from build123d import *

# Parameters (mm, degrees)
F0_R     = 10
F1_DEPTH = 25
F3_DEPTH = 12
F5_DEPTH = 25


with BuildPart() as f1:
    # F0 (on Top) → F1 (new body)
    with BuildSketch(Plane.XY):
        Circle(F0_R)
    extrude(amount=F1_DEPTH)

    # F2 (on face) → F3 (cut)
    with BuildSketch(Plane.XY.offset(25)):
        Polygon((2.886751, 5), (-2.886751, 5), (-5.773503, 0), (-2.886751, -5), (2.886751, -5), (5.773503, 0), align=None)
    extrude(amount=-F3_DEPTH, mode=Mode.SUBTRACT)

    # F4 (on face) → F5 (cut)
    with BuildSketch(Plane(origin=(0, 0, 0), x_dir=(1, 0, 0), z_dir=(0, 0, -1))):
        Polygon((1.057785, -4.400124), (4.400124, 1.057785), (-1.057785, 4.400124), (-4.400124, -1.057785), align=None)
    extrude(amount=-F5_DEPTH, mode=Mode.SUBTRACT)


solid = f1.part
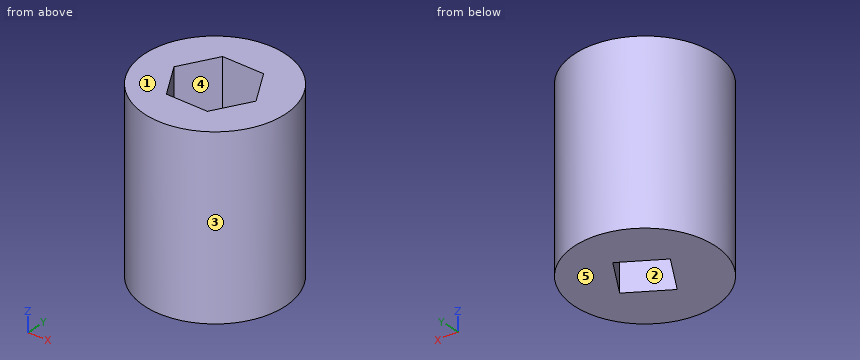
Work out the finished part from the listing and answer in its coordinate system (mm). Face numbers are marked on the shaded views. A direction names the side the tool comes from. Coordinates: 2 decimals unless noted, no trailing zeros. Write each loop counter-clockwise with the first axis right and the second up, starting at its lowest first coordinate (ties: lowest second). Pieces come first, ordered by that corner, then holes. Notation, with made-up numbers: (-8, 28.25) - (-2, 28.25) arc R22 cw to (-2, 59.25) - close; hole circle Ø5 at (-34.5, 89). An arc over 180 degrees is marked (long way). One line per question, with ' | ' between items.
1) For the marked faces 4 and 5, determine the directions among +Z, -Z, +X, -X, +Y, -Y from which every point of the face is accessible in a straight line to the end or side of a thin tool.
Checks:
face 4: +Z | face 5: -Z, +X, -X, +Y, -Y
2) Flat-ended cylindrical pins translate along their axes: P1, Ø1.5, axis at x = 2, z = 14, coming from the +Y side; P2, Ø2, axis at x = 7.5, z = 20, coming from the -Y side; P3, Ø10, axis at y = 5.5, z = 7, coming from the +X side. Find the tip coordinate at first contact, or state that the pin passes through.
Checks:
P1: y = 9.92 | P2: y = -7.6 | P3: x = 9.99
3) Consider probe 1 along Y at (x, z) = (-4.25, 3.75); probe 2 along X at (y, z) = (4, 10.75); probe 3 along X at (y, z) = (1.75, 8.75). Determine where each line is inside the solid, lowest interval first. Write a range as [from, to].
Checks:
probe 1: [-9.05, 0.81], [1.15, 9.05] | probe 2: [-9.17, 0.4], [1.3, 9.17] | probe 3: [-9.85, -3.27], [2.68, 9.85]
4) Find section D-D, the plane x = -5.25. Determine the outline of the cut face in (y, z).
Checks:
outline: (-8.51, 0) - (8.51, 0) - (8.51, 25) - (0.91, 25) - (0.91, 13) - (-0.91, 13) - (-0.91, 25) - (-8.51, 25) - close
5) Find section B-B, the plane z = 7.75. Determine the outline of the cut face in (x, y).
Checks:
outline: circle Ø20 at (0, 0); hole (-4.4, 1.06) - (-1.06, -4.4) - (4.4, -1.06) - (1.06, 4.4) - close
6) Find section A-A, the plane x = 3.5. Determine the outline of the cut face in (y, z).
Checks:
outline: (-9.37, 0) - (-1.61, 0) - (-1.61, 13) - (-3.94, 13) - (-3.94, 25) - (-9.37, 25) - close; (0.41, 0) - (9.37, 0) - (9.37, 25) - (3.94, 25) - (3.94, 13) - (0.41, 13) - close
7) The mould has two halves that part along Y. Classify the marked faces 1, 2 and 3: +Y half, -Y half, draft (parallel to the pull), parting line (faces both ways), or undercut.
Checks:
face 1: draft | face 2: undercut | face 3: parting line
8) Find section C-C, the plane y = 1.5. Determine the outline of the cut face in (x, z), and give its area (3 significant figures).
Checks:
outline: (-9.89, 0) - (-3.68, 0) - (-3.68, 13) - (-4.91, 13) - (-4.91, 25) - (-9.89, 25) - close; (2.83, 0) - (9.89, 0) - (9.89, 25) - (4.91, 25) - (4.91, 13) - (2.83, 13) - close | area: 292 mm2
